Part print with two shaded views. Sizes in mm from the minimum x, y, z corner. Round coordinates to 2 decimals unless told otherwise and drop trailing zeros. Loops run counter-clockwise (first coordinate to the right, second up) from the corner with the lowest first, then second, coordinate; pieces in that order, holes last. Notation, with made-up numbers: M -30.5,47 L 6.5,47 A11 ccw 6.5,66 Z; hole C -19.5,51.25 d7. An arc over 180 degrees is marked long. Use a Markdown table: item, result. Add a question column.
Item 1: Saw through at A-A on y = 32. Write the cut outline in (x, z), then the cut area to 3 significant figures.
Item 2: Saw through at B-B on x = 10. Write the cut outline in (y, z), then the cut area to 3 significant figures.
Item 3: Pin check, flat tips, straight feed: P1, Ø2.5, axis at x = 90, y = 32, coming from the -Z side; P2, Ø8, axis at x = 20.5, y = 18.5, coming from the -Z side. Stop position of each tip, or through.
Item 4: Saw through at D-D on x = 91. Write the cut outline in (y, z), then the cut area to 3 significant figures.
Item 5: Saw through at C-C on z = 3.2. Give the number of separate pieces and of enclosed holes in the cut face, then the cut area to 3 significant figures.
Item 6: Wall check: L1, parallel to Y at x = 10, z = 1.95; L2, parallel to X at y = 33, z = 2.15; L3, parallel to Y at x = 89.5, z = 1.05. Give the ranges that are in metal, low to high. Write a range as from..to.
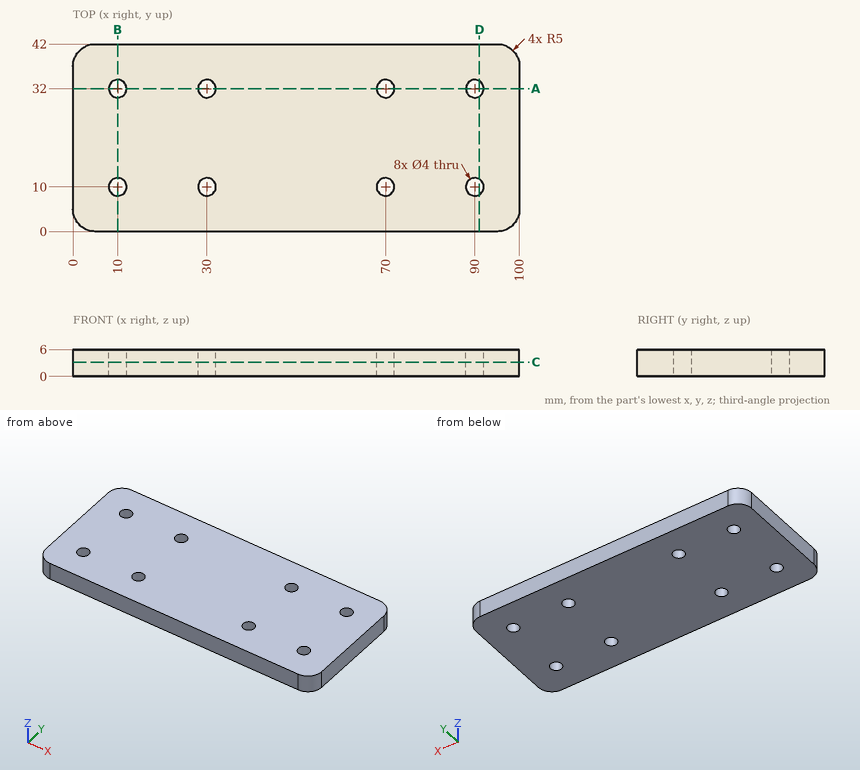
Entries:
| question | item | result |
|---|---|---|
| 1 | outline | M 0,0 L 8,0 L 8,6 L 0,6 Z; M 12,0 L 28,0 L 28,6 L 12,6 Z; M 32,0 L 68,0 L 68,6 L 32,6 Z; M 72,0 L 88,0 L 88,6 L 72,6 Z; M 92,0 L 100,0 L 100,6 L 92,6 Z |
| 1 | area | 504 mm2 |
| 2 | outline | M 0,0 L 8,0 L 8,6 L 0,6 Z; M 12,0 L 30,0 L 30,6 L 12,6 Z; M 34,0 L 42,0 L 42,6 L 34,6 Z |
| 2 | area | 204 mm2 |
| 3 | P1 | through |
| 3 | P2 | z = 0 |
| 4 | outline | M 0,0 L 8.27,0 L 8.27,6 L 0,6 Z; M 11.73,0 L 30.27,0 L 30.27,6 L 11.73,6 Z; M 33.73,0 L 42,0 L 42,6 L 33.73,6 Z |
| 4 | area | 210 mm2 |
| 5 | separate pieces | 1 |
| 5 | enclosed holes | 8 |
| 5 | area | 4,080 mm2 |
| 6 | L1 | 0..8, 12..30, 34..42 |
| 6 | L2 | 0..8.27, 11.73..28.27, 31.73..68.27, 71.73..88.27, 91.73..100 |
| 6 | L3 | 0..8.06, 11.94..30.06, 33.94..42 |
